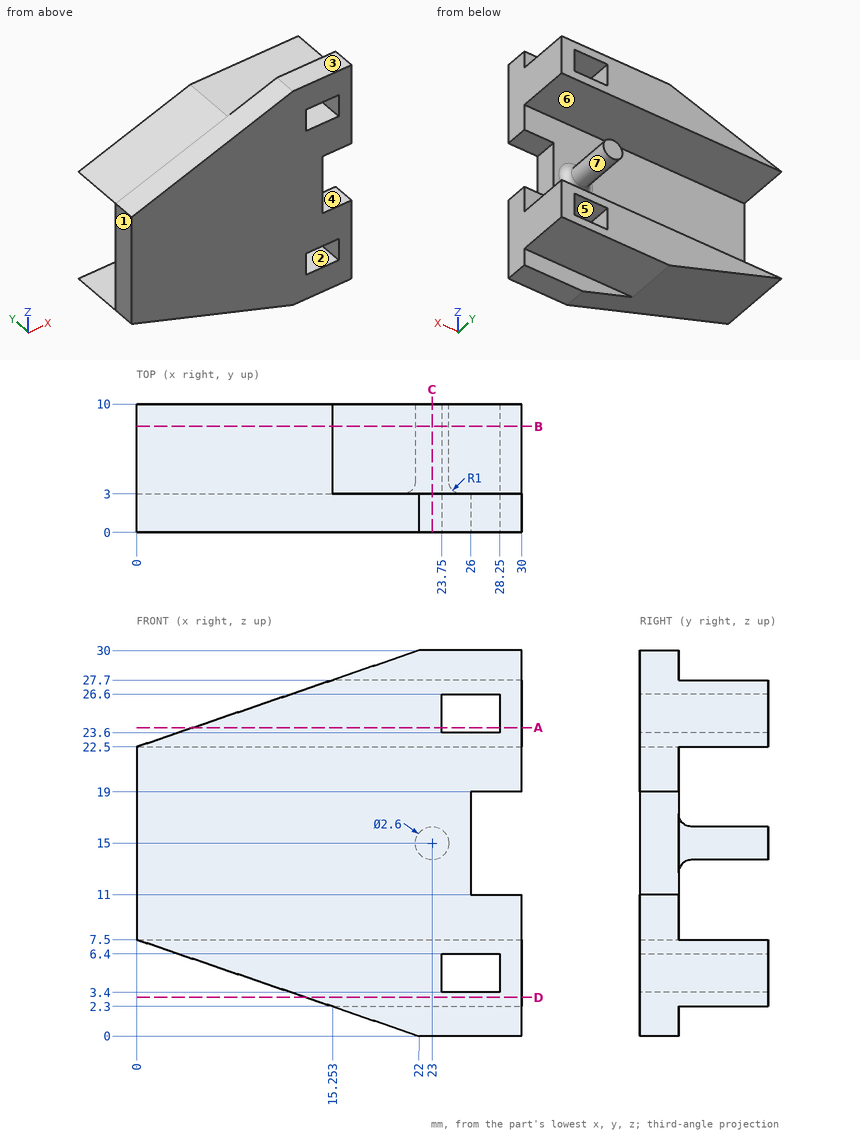
The drawing under review shows one solid part. Ordinate dimensions are in mm from its lowest x, y, z. A direction names the side the tool comes from. Round coordinates to 2 decimals unless told otherwise and drop trailing zeros. Loops run counter-clockwise (first coordinate to the right, second up) from the corner with the lowest first, then second, coordinate; pieces in that order, holes last.
Item 1: Take a section at A-A (z = 24). Write out the cut boundary in (x, y), then the cut area to 3 significant figures.
Determined:
outline: (4.4, 0) - (23.75, 0) - (23.75, 10) - (4.4, 10) - close; (28.25, 0) - (30, 0) - (30, 10) - (28.25, 10) - close
area: 211 mm2
Item 2: Take a section at C-C (x = 23). Write out the cut boundary in (y, z), then the cut area to 3 significant figures.
Determined:
outline: (0, 0) - (3, 0) - (3, 2.3) - (10, 2.3) - (10, 7.5) - (3, 7.5) - (3, 12.7) arc R1 cw to (4, 13.7) - (10, 13.7) - (10, 16.3) - (4, 16.3) arc R1 cw to (3, 17.3) - (3, 22.5) - (10, 22.5) - (10, 27.7) - (3, 27.7) - (3, 30) - (0, 30) - close
area: 181 mm2
Item 3: For line 1 (Z direction, x = 27.25, y = 3.5); line 2 (Z direction, x = 20.75, y = 6); line 3 (Y direction, x = 9, z = 16), list the stretches that pass through material, from the lowest coordinate up.
Determined:
line 1: z = 2.3 to 3.4, 6.4 to 7.5, 22.5 to 23.6, 26.6 to 27.7
line 2: z = 2.3 to 7.5, 22.5 to 27.7
line 3: y = 0 to 3
Item 4: Mouldability with a two-part tool opening along X and no side actions: class the marked faces 1, 2 and 3 as released by +X, released by -X, zero draft, split by the parting line, or undercut.
Determined:
face 1: released by -X
face 2: undercut
face 3: zero draft
Item 5: Clearance check with flat-ended pins moving along their axes: pin 1 Ø3 at (x, y) = (19.5, 7.5) entering from +Z; pin 2 Ø1.5 at (y, z) = (1, 13.5) entering from +X; pin 3 Ø3.5 at (x, y) = (24.5, 6.5) entering from -Z. State where each tip first meets the part, or that it passes through.
Determined:
pin 1: stops at z = 27.7
pin 2: stops at x = 26
pin 3: stops at z = 2.3
Item 6: Take a section at D-D (z = 3). Write out the cut boundary in (x, y), then the cut area to 3 significant figures.
Determined:
outline: (13.2, 0) - (30, 0) - (30, 10) - (13.2, 10) - close
area: 168 mm2
Item 7: For the marked faces 4, 5, 6 and 7, list the 3-axis set-ups (+Z, -Z, +X, -X, +Y, -Y) from which the entire face can be reached by the end or side of a thin tool; tool diameter is ignored.
Determined:
face 4: +X, +Y, -Y
face 5: +Y, -Y
face 6: +X, -X, +Y
face 7: +Y
Item 8: Take a section at B-B (y = 8.25). Write out the cut boundary in (x, z).
Determined:
outline: (0, 7.5) - (15.25, 2.3) - (30, 2.3) - (30, 7.5) - close; (0, 22.5) - (30, 22.5) - (30, 27.7) - (15.25, 27.7) - close; circle Ø2.6 at (23, 15); hole (23.75, 3.4) - (28.25, 3.4) - (28.25, 6.4) - (23.75, 6.4) - close; hole (23.75, 23.6) - (28.25, 23.6) - (28.25, 26.6) - (23.75, 26.6) - close
